Autodesk Inventor part; units mm, degrees
ref_plane "YZ Plane" through (0, 0, 0) normal (1, 0, 0) x (0, 1, 0)
ref_plane "XZ Plane" through (0, 0, 0) normal (0, 1, 0) x (-1, 0, 0)
ref_plane "XY Plane" through (0, 0, 0) normal (0, 0, 1) x (1, 0, 0)
sketch "Sketch1" plane through (0, 0, 0) normal (0, 0, 1) x (1, 0, 0)
  circle A0 centre (0, 0) radius 1.4224
  circle A1 centre (0, 0) radius 3.175
  line L0 (0, 0) -> (-15.875, 0) construction
  circle A2 centre (-2.0016, -10.9307) radius 3.175
  circle A3 centre (-2.0016, -10.9307) radius 5 construction
  circle A4 centre (-2.0016, -10.9307) radius 1.5
  line L1 (0, 0) -> (-2.0016, -10.9307) construction
  line L2 (-2.0016, -10.9307) -> (-3.4771, -10.6606) construction
  line L3 (0, 0) -> (-2.0016, -10.9307) construction
  arc A5 (-5.0684, -10.109) -> (1.0652, -11.7525) centre (-2.0016, -10.9307) ccw
  arc A6 (-1.2212, -2.9308) -> (-15.875, 0) centre (-15.875, -38.1) ccw
  arc A7 (-15.875, 3.175) -> (-15.875, 0) centre (-15.875, 1.5875) ccw
  line L4 (-15.875, 3.175) -> (0, 3.175)
  line L5 (-2.0016, -10.9307) -> (-4.9305, 0) construction
  line L6 (1.0652, -10.109) -> (-1.8637, 0.8218)
  line L7 (-7.9973, -0.8218) -> (-5.0684, -11.7525)
  arc A8 (-5.0684, -11.7525) -> (1.0652, -10.109) centre (-2.0016, -10.9307) ccw
  arc A9 (-1.8637, 0.8218) -> (-7.9973, -0.8218) centre (-4.9305, 0) ccw
  circle A10 centre (6.7469, -0.7937) radius 3.175
  circle A11 centre (6.7469, -0.7937) radius 1.5
  line L8 (7.1178, 2.3595) -> (0.371, 3.1533)
  arc A12 (4.6726, -3.1975) -> (-0.0011, -6.1296) centre (2.7869, -5.3826) ccw
  circle A13 centre (6.7469, -0.7937) radius 5 construction
  point P0 (-5.0684, -10.109)
  point P1 (0, 3.175)
  point P2 (-7.9969, -0.8234)
  point P3 (1.0652, -10.109)
  point P4 (-0.8218, -3.0668)
  point P5 (-2.4653, 2.0008)
  point P6 (0.6312, -3.1116)
  point P7 (1.4598, -2.8195)
  point P8 (-1.4243, -1.0642)
  point P9 (-1.7024, 0.5129)
  point P10 (1.0652, -10.109)
  point P11 (-5.0684, -11.7525)
  dimension "d24" = 3
  dimension "d0" = 2.8448
  dimension "d1" = 6.35
  dimension "d9" = 15.875
  dimension "d22" = 6.35
  dimension "d23" = 10
  dimension "Arm_Length" = 11.1125
  dimension "d29" = 3.175
  dimension "d30" = 6.35
  dimension "d31" = 6.35
  dimension "d32" = 3
  dimension "d36" = 10
  dimension "Arm_Angle" = 105
  dimension "d38" = 4.7625
  dimension "d39" = 6.7469
  dimension "d40" = 0.7937
extrude "Extrusion1" add sketch "Sketch1" along normal blind 3.048
fillet "Fillet1" radius 3.175 1 edges at (-7.9969, -0.8234, 1.524)
properties part number "Lever" material "Aluminum 6061"
Source: CAD feature listing. Evaluate the final solid. Frame: model axes, mm. A direction names the side the tool comes from. Give positions to 0.01 mm unless a question says otherwise; leave off trailing zeros. Order: outer loops, then holes, each group sorted by start corner. A loop starts at its lowest first (then second) coordinate and runs counter-clockwise, first axis right, second up. Notation, with made-up numbers: (7, 17.5) -> (17, 17.5) arc R20 ccw to (17, 37.5) -> close; hole circle Ø7 at (64, 8). An arc over 180 degrees is marked (long way). Write item = value, one per line.
Q1. Cut plane D-D, the plane x = -7.75. Output: boundary loops of the cut face in (y, z) (3 decimals).
Data:
outline = (-2.076, 0) -> (3.175, 0) -> (3.175, 3.048) -> (-2.076, 3.048) -> close
Q2. Set-up query: faces 1 (the face through (3.79, 2.75, 1.5)), 2 (the face through (0.54, -8.15, 1.5)). Return all of +Z, -Z, +X, -X, +Y, -Y with unobstructed straight access to the full face (end or side cutting, diameter ignored); none if empty.
Data:
face_1 = +Z, -Z, +X, +Y
face_2 = +Z, -Z, +X
Q3. Cut plane C-C, the plane y = -9.75. Output: boundary loops of the cut face in (x, z), and give its area (3 significant figures).
Data:
outline = (-5.6, 0) -> (-2.93, 0) -> (-2.93, 3.05) -> (-5.6, 3.05) -> close; (-1.08, 0) -> (0.97, 0) -> (0.97, 3.05) -> (-1.08, 3.05) -> close
area = 14.4 mm^2
Q4. Pull-direction query (Y, two-part tool) for faces 3 (the face through (-17.462, 1.553, 1.503)), 4 (the face through (8.18, -1.24, 1.5)), 5 (the face through (-6.29, -7.19, 1.5)); classes: released by +Y, released by -Y, zero draft, split by the parting line, or undercut.
Data:
face_3 = split by the parting line
face_4 = undercut
face_5 = released by -Y
Q5. Cut plane A-A, the plane y = -2. Output: boundary loops of the cut face in (x, z).
Data:
outline = (-7.79, 0) -> (5.86, 0) -> (5.86, 3.05) -> (-7.79, 3.05) -> close; (7.64, 0) -> (9.68, 0) -> (9.68, 3.05) -> (7.64, 3.05) -> close
Q6. Pin query (flat end, axial travel): pin 1 (3.5 mm diameter, centred on x = 0, y = 0, fed in from +Z); pin 2 (2.5 mm diameter, centred on x = 6.75, y = -0.79, fed in from +Z). Return the tip coordinate at first contact, or that it passes through.
Data:
pin_1 = 3.05
pin_2 = through
Q7. Material intervals for line 1 (X direction, y = 0.5, z = 1.2); line 2 (Y direction, x = 6.5, z = 2.05); line 3 (X direction, y = -1, z = 2.6), sorted ascending. Write a range as from..to.
Data:
line_1 = -17.03..-1.33, 1.33..5.99, 7.51..9.65
line_2 = -3.96..-2.27, 0.69..2.43
line_3 = -8.7..-1.01, 1.01..5.26, 8.23..9.92
Q8. Cut plane B-B, the plane z = 2. State how many separate pieces and enclosed holes the cut face has, and give its area (3 significant figures).
Data:
separate_pieces = 1
enclosed_holes = 3
area = 185 mm^2
